```python
from build123d import *

# Parameters (mm, degrees)
BOSS_EXTRUDE1_DEPTH = 1.59
SKETCH2_R           = 2.5
SKETCH2_R_2         = 1.75
CUT_EXTRUDE2_DEPTH  = 1.59
SKETCH3_W           = 1.59
SKETCH3_H           = 40.336400608
BOSS_EXTRUDE2_DEPTH = 30.602
SKETCH5_R           = 2.5
SKETCH5_R_2         = 1.75
CUT_EXTRUDE4_DEPTH  = 10
SKETCH6_W           = 32.192
SKETCH6_H           = 10
BOSS_EXTRUDE3_DEPTH = 1.59
SKETCH7_R           = 1.75
CUT_EXTRUDE5_DEPTH  = 10
SKETCH8_R           = 1.25
CUT_EXTRUDE6_DEPTH  = 10


with BuildPart() as part:
    # Sketch1 → Boss-Extrude1 (new body)
    with BuildSketch(Plane.XY):
        with BuildLine():
            Line((-39.610035237, 20.168200304), (39.610035237, 20.168200304))
            ThreePointArc((39.610035237, 20.168200304), (59.77823554, 0), (39.610035237, -20.168200304))
            Line((39.610035237, -20.168200304), (-39.610035237, -20.168200304))
            Line((-39.610035237, -20.168200304), (-99.729964763, -20.168200304))
            Line((-99.729964763, -20.168200304), (-99.729964763, 20.168200304))
            Line((-99.729964763, 20.168200304), (-39.610035237, 20.168200304))
        make_face()
    extrude(amount=BOSS_EXTRUDE1_DEPTH)

    # Sketch2 → Cut-Extrude2 (cut)
    with BuildSketch(Plane.XY.offset(1.59)):
        with Locations((39.610035237, 0)):
            Circle(SKETCH2_R)
        with Locations((48.110035237, 0)):
            Circle(SKETCH2_R_2)
        with Locations((18.360035237, 0)):
            Circle(SKETCH2_R_2)
        with Locations((-11.639964763, 0)):
            Circle(SKETCH2_R_2)
        with Locations((-41.389964763, 0)):
            Circle(SKETCH2_R_2)
    extrude(amount=-CUT_EXTRUDE2_DEPTH, mode=Mode.SUBTRACT)

    # Sketch3 → Boss-Extrude2 (add)
    with BuildSketch(Plane.XY.offset(1.59)):
        with Locations((-98.934964763, 0)):
            Rectangle(SKETCH3_W, SKETCH3_H)
    extrude(amount=BOSS_EXTRUDE2_DEPTH)

    # Sketch5 → Cut-Extrude4 (cut)
    with BuildSketch(Plane.ZY.offset(99.729964763)):
        with Locations((16.096, 0)):
            Circle(SKETCH5_R)
        with Locations((16.096, 8.5)):
            Circle(SKETCH5_R_2)
        with Locations((16.096, -21.25)):
            Circle(SKETCH5_R_2)
    extrude(amount=-CUT_EXTRUDE4_DEPTH, mode=Mode.SUBTRACT)

    # Sketch6 → Boss-Extrude3 (add)
    with BuildSketch(Plane.ZY.offset(99.729964763)):
        with Locations((16.096, -25.168200304)):
            Rectangle(SKETCH6_W, SKETCH6_H)
    extrude(amount=-BOSS_EXTRUDE3_DEPTH)

    # Sketch7 → Cut-Extrude5 (cut)
    with BuildSketch(Plane.ZY.offset(99.729964763)):
        with Locations((16.096, -21.25)):
            Circle(SKETCH7_R)
    extrude(amount=-CUT_EXTRUDE5_DEPTH, mode=Mode.SUBTRACT)

    # Sketch8 → Cut-Extrude6 (cut)
    with BuildSketch(Plane.XY.offset(1.59)):
        with Locations((-73.139964763, 0)):
            Circle(SKETCH8_R)
    extrude(amount=-CUT_EXTRUDE6_DEPTH, mode=Mode.SUBTRACT)


solid = part.part
```
The listing builds one solid part. Answer for the finished solid, in the listing's coordinates (mm). A direction names the side the tool comes from. Coordinates: 2 decimals unless noted, no trailing zeros. Write each loop counter-clockwise with the first axis right and the second up, starting at its lowest first coordinate (ties: lowest second). Pieces come first, ordered by that corner, then holes. Notation, with made-up numbers: (76, -27.75) - (92, -27.75) arc R20 ccw to (92, 8.25) - close; hole circle Ø1 at (-39, -5.5). An arc over 180 degrees is marked (long way). Return JSON: item names as keys, results as strings. Group by question number.
Q1. Flat-ended cylindrical pins translate along their axes: pin 1 Ø4 at (x, y) = (48.11, 0) entering from +Z; pin 2 Ø1 at (y, z) = (14, 15) entering from +X; pin 3 Ø1.7 at (x, z) = (-41, 1) entering from -Y. Find the tip coordinate at first contact, or state that the pin passes through.
Q2. Which of the six approach directions +Z, -Z, +X, -X, +Y, -Y give full straight-line access (tool end or side, diameter ignored) to faces 1 (the flat face through (-18, 0, 1.59)), 2 (the cylindrical face through (49.727, -0.67, 0.806))?
Q3. For a pull along Z with two mould halves and no side action, classify faces 3 (the flat face through (-21, 0, 0)), 4 (the cylindrical face through (-98.9, 0.1, 13.6)), 5 (the cylindrical face through (59.773, 0.443, 0.784)) as +Z half, -Z half, draft (parallel to the pull), parting line (faces both ways), or undercut.
Q4. The part is cut by section C-C on z = 22. Write down the section's boundary in (x, y), and give its area (3 significant figures).
Q5. The part is cut by section B-B on x = 13.5. Write down the section's boundary in (y, z), and give its area (3 significant figures).
Q6. Find the intervals of material crossed by line 1 along Z through (x, y) = (-25.5, -10.5); line 2 along X through (y, z) = (-11, 10), in increasing order. Write a range as [from, to].
Q7. The part is cut by section A-A on y = 8.5. Write down the section's boundary in (x, z).
Evaluation:
{
 "1": {"pin 1": "stops at z = 1.59", "pin 2": "stops at x = -98.14", "pin 3": "stops at y = -20.17"},
 "2": {"face 1": "+Z, +X, +Y, -Y", "face 2": "+Z, -Z"},
 "3": {"face 3": "-Z half", "face 4": "undercut", "face 5": "draft"},
 "4": {"outline": "(-99.73, -30.17) - (-98.14, -30.17) - (-98.14, 20.17) - (-99.73, 20.17) - close", "area": "80.0 mm2"},
 "5": {"outline": "(-20.17, 0) - (20.17, 0) - (20.17, 1.59) - (-20.17, 1.59) - close", "area": "64.1 mm2"},
 "6": {"line 1": "z = [0, 1.59]", "line 2": "x = [-99.73, -98.14]"},
 "7": {"outline": "(-99.73, 0) - (57.9, 0) - (57.9, 1.59) - (-98.14, 1.59) - (-98.14, 14.35) - (-99.73, 14.35) - close; (-99.73, 17.85) - (-98.14, 17.85) - (-98.14, 32.19) - (-99.73, 32.19) - close"}
}
